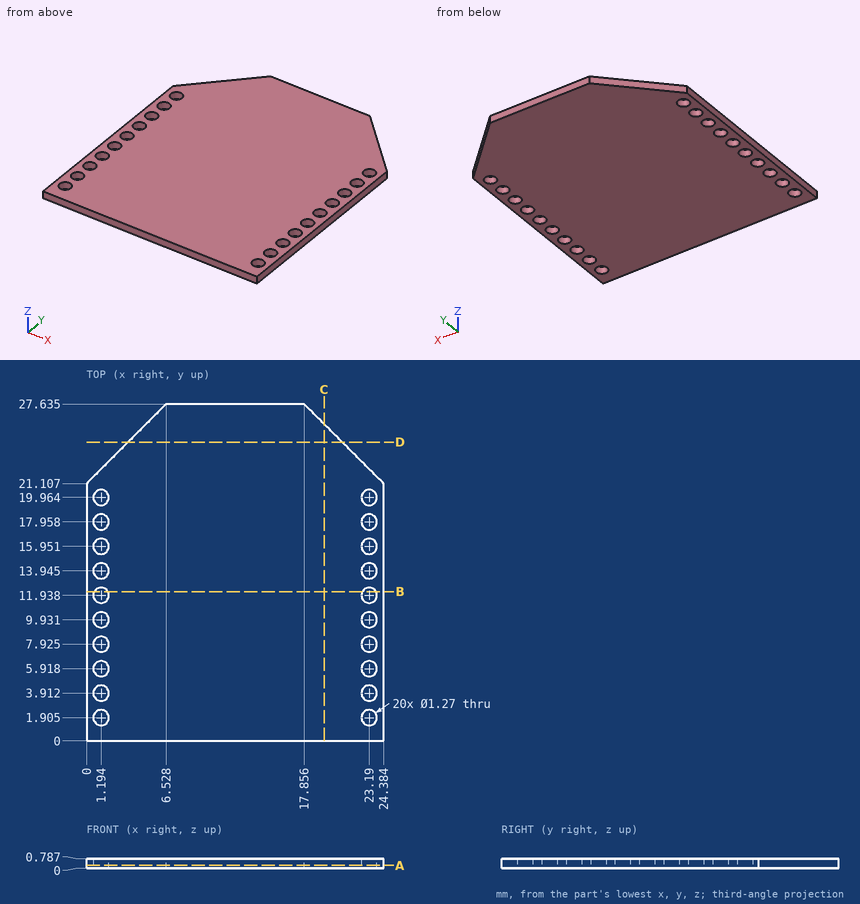
Answer from the drawing. Dimensions are ordinates in mm from the lowest x, y and z of the part. Give positions to 0.01 mm unless a question says otherwise; leave off trailing zeros. Order: outer loops, then holes, each group sorted by start corner. A loop starts at its lowest first (then second) coordinate and runs counter-clockwise, first axis right, second up.
Item 1: The part is cut by section C-C, the plane x = 19.5. Give the vertices of the cut face in (y, z).
From the geometry:
outline: (0, 0) - (25.99, 0) - (25.99, 0.79) - (0, 0.79) - close
Item 2: The part is cut by section B-B, the plane y = 12.25. Give the vertices of the cut face in (x, z).
From the geometry:
outline: (0, 0) - (0.64, 0) - (0.64, 0.79) - (0, 0.79) - close; (1.75, 0) - (22.64, 0) - (22.64, 0.79) - (1.75, 0.79) - close; (23.74, 0) - (24.38, 0) - (24.38, 0.79) - (23.74, 0.79) - close
Item 3: The part is cut by section D-D, the plane y = 24.5. Give the vertices of the cut face in (x, z).
From the geometry:
outline: (3.39, 0) - (20.99, 0) - (20.99, 0.79) - (3.39, 0.79) - close
Item 4: The part is cut by section A-A, the plane z = 0.25. Count the separate pieces of the cut face and the enclosed holes in it, and give its area (3 significant figures).
From the geometry:
separate pieces: 1
enclosed holes: 20
area: 606 mm2
Item 5: Find the intervals of material crossed by probe 1 along X at (y, z) = (14, 0.15); probe 2 along X at (y, z) = (18.5, 0.3) (1 decimal); probe 3 along X at (y, z) = (24.75, 0.4) (1 decimal), in increasing order.
From the geometry:
probe 1: x = 0 to 0.56, 1.83 to 22.56, 23.82 to 24.38
probe 2: x = 0 to 0.9, 1.5 to 22.9, 23.5 to 24.4
probe 3: x = 3.6 to 20.7
